from build123d import *

# Parameters (mm, degrees)
CUT_EXTRUDE1_DEPTH      = 12
CUT_EXTRUDE1_DEPTH_BACK = 2
BOSS_EXTRUDE1_DEPTH     = 1
CIRPATTERN4_COUNT       = 4


with BuildPart() as part:
    # Sketch1 → Revolve1 (revolve)
    with BuildSketch(Plane(origin=(0, 0, 0), x_dir=(1, 0, 0), z_dir=(0, 1, 0))):
        with BuildLine():
            Line((8.5, 7.032838072), (8.5, 2.5))
            ThreePointArc((8.5, 2.5), (7.621320344, 0.378679656), (5.5, -0.5))
            Line((5.5, -0.5), (0, -0.5))
            Line((0, -0.5), (0, 0.5))
            Line((0, 0.5), (5.5, 0.5))
            ThreePointArc((5.5, 0.5), (6.914213562, 1.085786438), (7.5, 2.5))
            Line((7.5, 2.5), (7.5, 11.5))
            Line((7.5, 11.5), (8.5, 11.5))
            Line((8.5, 11.5), (8.5, 7.032838072))
        make_face()
    revolve(axis=Axis((12.5, 0, 0), (0, 0, -1)))

    # Sketch2 → Cut-Extrude1 (cut, two sides)
    with BuildSketch(Plane(origin=(0, 0, -0.5), x_dir=(-1, 0, 0), z_dir=(0, 0, -1))) as cut_extrude1_sk:
        with BuildLine():
            Line((-3.5, 8.674675786), (-3.5, 3))
            Line((-3.5, 3), (-0.3653389, 3))
            ThreePointArc((-0.3653389, 3), (-1.558383974, 6.044091225), (-3.5, 8.674675786))
        make_face()
        with BuildLine():
            Line((-3.825324214, -9), (-9.5, -9))
            Line((-9.5, -9), (-9.5, -12.1346611))
            ThreePointArc((-9.5, -12.1346611), (-6.455908775, -10.941616026), (-3.825324214, -9))
        make_face()
        with BuildLine():
            Line((-21.5, -8.674675786), (-21.5, -3))
            Line((-21.5, -3), (-24.6346611, -3))
            ThreePointArc((-24.6346611, -3), (-23.441616026, -6.044091225), (-21.5, -8.674675786))
        make_face()
        with BuildLine():
            Line((-21.174675786, 9), (-15.5, 9))
            Line((-15.5, 9), (-15.5, 12.1346611))
            ThreePointArc((-15.5, 12.1346611), (-18.544091225, 10.941616026), (-21.174675786, 9))
        make_face()
    extrude(amount=CUT_EXTRUDE1_DEPTH, mode=Mode.SUBTRACT)
    extrude(cut_extrude1_sk.sketch, amount=-CUT_EXTRUDE1_DEPTH_BACK, mode=Mode.SUBTRACT)

    # Sketch3 → Boss-Extrude1 (add)
    with BuildSketch(Plane(origin=(0, 3, 0), x_dir=(1, 0, 0), z_dir=(0, 1, 0))):
        with BuildLine():
            Line((0.3653389, 0.5), (3.5, 0.5))
            Line((3.5, 0.5), (3.5, 9.5))
            ThreePointArc((3.5, 9.5), (1.171429987, 5.265136415), (0.3653389, 0.5))
        make_face()
        with BuildLine():
            Line((3.5, -0.5), (3.5, 0.5))
            Line((3.5, 0.5), (0.3653389, 0.5))
            ThreePointArc((0.3653389, 0.5), (0.373979974, -0.000298405), (0.399892887, -0.5))
            Line((0.399892887, -0.5), (3.5, -0.5))
        make_face()
    boss_extrude1 = extrude(amount=BOSS_EXTRUDE1_DEPTH)

    # CirPattern4: Boss-Extrude1 ×4 about axis
    cirpattern4_axis = Axis((12.5, 0, 0), (0, 0, 1))
    for i in range(1, CIRPATTERN4_COUNT):
        add(boss_extrude1.rotate(cirpattern4_axis, i * 360 / CIRPATTERN4_COUNT))


solid = part.part
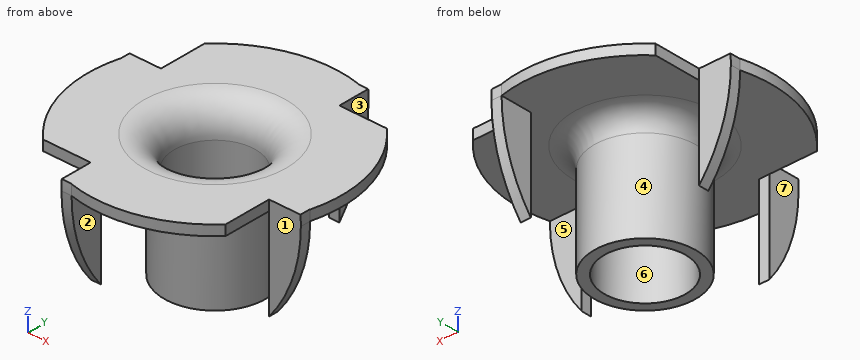
CAD build for the part. Positions are in the model's coordinates, mm. Face numbers are marked on the shaded views. A direction names the side the tool comes from. Give positions to 0.01 mm unless a question says otherwise; leave off trailing zeros. Order: outer loops, then holes, each group sorted by start corner. A loop starts at its lowest first (then second) coordinate and runs counter-clockwise, first axis right, second up. Notation, with made-up numbers: (-1.75, 86.25) -> (33.25, 86.25) arc R9 ccw to (33.25, 90.25) -> close; hole circle Ø2 at (83, 55). An arc over 180 degrees is marked (long way). Return JSON: item names as keys, results as strings.
Q1. Saw through at A-A (x = 12.5). Write the cut outline in (y, z).
Working result:
{"outline": "(-12.5, -0.5) -> (-7, -0.5) arc R2 cw to (-5, -2.5) -> (-5, -11.5) -> (-4, -11.5) -> (-4, -2.5) arc R3 ccw to (-7, 0.5) -> (-12.5, 0.5) -> close; (4, -11.5) -> (5, -11.5) -> (5, -2.5) arc R2 cw to (7, -0.5) -> (12.5, -0.5) -> (12.5, 0.5) -> (7, 0.5) arc R3 ccw to (4, -2.5) -> close"}
Q2. Mould opens along Y. For the marked faces 5, 6 and 7 say: pulls with the +Y half, pulls with the -Y half, needs draft (parallel to the pull), parting line crosses it, or undercut.
Working result:
{"face 5": "pulls with the +Y half", "face 6": "undercut", "face 7": "needs draft"}
Q3. Saw through at D-D (z = -1.5). Write the cut outline in (x, y).
Working result:
{"outline": "(0.4, 3) -> (3.5, 3) -> (3.5, 4) -> (0.4, 4) -> close; circle Ø10.54 at (12.5, 0); (8.5, -12.1) -> (9.5, -12.1) -> (9.5, -9) -> (8.5, -9) -> close; (15.5, 9) -> (16.5, 9) -> (16.5, 12.1) -> (15.5, 12.1) -> close; (21.5, -4) -> (24.6, -4) -> (24.6, -3) -> (21.5, -3) -> close; hole circle Ø8.34 at (12.5, 0)"}
Q4. Which spindle directions (+Z, -Z, +X, -X, +Y, -Y) get a long thin tool onto all of the face, cutting with end or side? Do the marked faces 1, 2, 3 and 4. Say none if no direction does.
Working result:
{"face 1": "+Z, -Z, +X, -Y", "face 2": "-Z, +X, -Y", "face 3": "+Z, -Z, +X, +Y", "face 4": "-Z"}
Q5. Saw through at C-C (z = -8.5). Write the cut outline in (x, y).
Working result:
{"outline": "(2.77, 3) -> (3.5, 3) -> (3.5, 4) -> (2.77, 4) -> close; circle Ø10 at (12.5, 0); (8.5, -9.73) -> (9.5, -9.73) -> (9.5, -9) -> (8.5, -9) -> close; (15.5, 9) -> (16.5, 9) -> (16.5, 9.73) -> (15.5, 9.73) -> close; (21.5, -4) -> (22.23, -4) -> (22.23, -3) -> (21.5, -3) -> close; hole circle Ø8 at (12.5, 0)"}
Q6. Saw through at B-B (y = 0). Write the cut outline in (x, z).
Working result:
{"outline": "(0, -0.5) -> (5.5, -0.5) arc R2 cw to (7.5, -2.5) -> (7.5, -11.5) -> (8.5, -11.5) -> (8.5, -2.5) arc R3 ccw to (5.5, 0.5) -> (0, 0.5) -> close; (16.5, -11.5) -> (17.5, -11.5) -> (17.5, -2.5) arc R2 cw to (19.5, -0.5) -> (25, -0.5) -> (25, 0.5) -> (19.5, 0.5) arc R3 ccw to (16.5, -2.5) -> close"}
Q7. Flat gauge pins, fed straight in: pin 1 (3 mm diameter, centred on y = -8.5, z = -8.5, fed in from +X); pin 2 (1.5 mm diameter, centred on x = 16, z = -7, fed in from -Y); pin 3 (0.8 mm diameter, centred on y = -7, z = 0, fed in from +X); pin 4 (5 mm diameter, centred on x = 12.5, y = 0, fed in from -Z). Where does each tip first touch, or does it go through?
Working result:
{"pin 1": "x = 9.5", "pin 2": "y = -4.18", "pin 3": "x = 21.5", "pin 4": "through"}
Q8. Drill centre lines: line 1 (X direction, y = 3.5, z = -4); line 2 (Y direction, x = 12.5, z = -5); line 3 (Z direction, x = 18.75, y = 4.75). Where is each one in solid material? Low to high.
Working result:
{"line 1": "0.79 to 3.5, 8.93 to 10.56, 14.44 to 16.07", "line 2": "-5 to -4, 4 to 5", "line 3": "-0.5 to 0.5"}
